For this review, take the finished solid that the model builds, in its own axes (mm). Give positions to 0.01 mm unless a question says otherwise; leave off trailing zeros. Loops run counter-clockwise (first coordinate to the right, second up) from the corner with the lowest first, then second, coordinate; pieces in that order, holes last. Notation, with made-up numbers: (30.25, 41) - (66.25, 41) arc R28 cw to (66.25, 69) - close; hole circle Ø5 at (-24, 14). An arc over 180 degrees is marked (long way). Put each result on its own line as item: value.
Autodesk Inventor part; units mm, degrees
ref_plane "YZ Plane" through (0, 0, 0) normal (1, 0, 0) x (0, 1, 0)
ref_plane "XZ Plane" through (0, 0, 0) normal (0, 1, 0) x (-1, 0, 0)
ref_plane "XY Plane" through (0, 0, 0) normal (0, 0, 1) x (1, 0, 0)
sketch "Sketch1" plane through (0, 0, 0) normal (0, 0, 1) x (1, 0, 0)
  line L0 (-101.9973, -32.9991) -> (101.9973, -32.9991)
  line L1 (-101.9973, 33.0009) -> (101.9973, 33.0009)
  line L2 (-103.9973, -30.9991) -> (-103.9973, 31.0009)
  line L3 (103.9973, 31.0009) -> (103.9973, -30.9991)
  arc A0 (-103.9973, -30.9991) -> (-101.9973, -32.9991) centre (-101.9973, -30.9991) ccw
  arc A1 (101.9973, -32.9991) -> (103.9973, -30.9991) centre (101.9973, -30.9991) ccw
  line L4 (103.9973, 31.0009) -> (103.9973, 33.0009)
  line L5 (101.9973, 33.0009) -> (103.9973, 33.0009)
  line L6 (-103.9973, 31.0009) -> (-103.9973, 33.0009)
  line L7 (-101.9973, 33.0009) -> (-103.9973, 33.0009)
  line L8 (57.998, 18.2189) -> (41.998, 18.2189)
  line L9 (41.998, 13.2189) -> (57.998, 13.2189)
  line L10 (-58.002, 18.2189) -> (-42.002, 18.2189)
  line L11 (-42.002, 13.2189) -> (-58.002, 13.2189)
  line L12 (32.998, 18.2189) -> (-33.002, 18.2189)
  line L13 (-33.002, 13.2189) -> (32.998, 13.2189)
  arc A2 (34.998, 16.2189) -> (32.998, 18.2189) centre (32.998, 16.2189) ccw
  arc A3 (-35.002, 15.2189) -> (-33.002, 13.2189) centre (-33.002, 15.2189) ccw
  arc A4 (-33.002, 18.2189) -> (-35.002, 16.2189) centre (-33.002, 16.2189) ccw
  arc A5 (-40.002, 16.2189) -> (-42.002, 18.2189) centre (-42.002, 16.2189) ccw
  arc A6 (-42.002, 13.2189) -> (-40.002, 15.2189) centre (-42.002, 15.2189) ccw
  arc A7 (-60.002, 15.2189) -> (-58.002, 13.2189) centre (-58.002, 15.2189) ccw
  arc A8 (-58.002, 18.2189) -> (-60.002, 16.2189) centre (-58.002, 16.2189) ccw
  arc A9 (39.998, 15.2189) -> (41.998, 13.2189) centre (41.998, 15.2189) ccw
  arc A10 (41.998, 18.2189) -> (39.998, 16.2189) centre (41.998, 16.2189) ccw
  arc A11 (59.998, 16.2189) -> (57.998, 18.2189) centre (57.998, 16.2189) ccw
  arc A12 (57.998, 13.2189) -> (59.998, 15.2189) centre (57.998, 15.2189) ccw
  arc A13 (32.998, 13.2189) -> (34.998, 15.2189) centre (32.998, 15.2189) ccw
  line L14 (59.998, 16.2189) -> (39.998, 16.2189)
  line L15 (39.998, 15.2189) -> (59.998, 15.2189)
  line L16 (34.998, 16.2189) -> (-35.002, 16.2189)
  line L17 (-35.002, 15.2189) -> (34.998, 15.2189)
  line L18 (-40.002, 16.2189) -> (-60.002, 16.2189)
  line L19 (-60.002, 15.2189) -> (-40.002, 15.2189)
  circle A14 centre (-59.9992, -3) radius 2
  circle A15 centre (59.9979, -3) radius 2
  line L20 (93.998, -24.9998) -> (93.998, -10.0006)
  line L21 (93.998, -10.0006) -> (98.998, -10.0006)
  line L22 (98.998, -24.9998) -> (98.998, -10.0006)
  line L23 (93.998, -24.9998) -> (98.998, -24.9998)
  line L24 (93.998, 9.9994) -> (93.998, 25.0009)
  line L25 (93.998, 25.0009) -> (98.998, 25.0009)
  line L26 (98.998, 9.9994) -> (98.998, 25.0009)
  line L27 (93.998, 9.9994) -> (98.998, 9.9994)
  line L28 (87.498, 20.0009) -> (57.498, 20.0009)
  line L29 (57.498, 20.0009) -> (57.498, 25.0009)
  line L30 (87.498, 25.0009) -> (57.498, 25.0009)
  line L31 (87.498, 20.0009) -> (87.498, 25.0009)
  line L32 (27.498, 20.0009) -> (-27.502, 20.0009)
  line L33 (-27.502, 20.0009) -> (-27.502, 25.0009)
  line L34 (27.498, 25.0009) -> (-27.502, 25.0009)
  line L35 (27.498, 20.0009) -> (27.498, 25.0009)
  line L36 (-57.502, 20.0009) -> (-87.502, 20.0009)
  line L37 (-87.502, 20.0009) -> (-87.502, 25.0009)
  line L38 (-57.502, 25.0009) -> (-87.502, 25.0009)
  line L39 (-57.502, 20.0009) -> (-57.502, 25.0009)
  line L40 (-99.002, 9.9994) -> (-99.002, 25.0009)
  line L41 (-99.002, 25.0009) -> (-94.002, 25.0009)
  line L42 (-94.002, 9.9994) -> (-94.002, 25.0009)
  line L43 (-99.002, 9.9994) -> (-94.002, 9.9994)
  line L44 (-99.002, -24.9998) -> (-99.002, -10.0006)
  line L45 (-99.002, -10.0006) -> (-94.002, -10.0006)
  line L46 (-94.002, -24.9998) -> (-94.002, -10.0006)
  line L47 (-99.002, -24.9998) -> (-94.002, -24.9998)
  point P0 (-85.2166, -15.942)
  point P1 (-103.9973, -32.9991)
  point P2 (103.9973, -32.9991)
  point P3 (59.998, 18.2189)
  point P4 (59.998, 13.2189)
  point P5 (-60.002, 16.2189)
  point P6 (59.998, 15.2189)
  point P7 (59.9979, -3)
extrude "Extrusion1" add sketch "Sketch1" along normal blind 5
properties part number "case bottom front" material "Nylon, molybdenum disulphide"
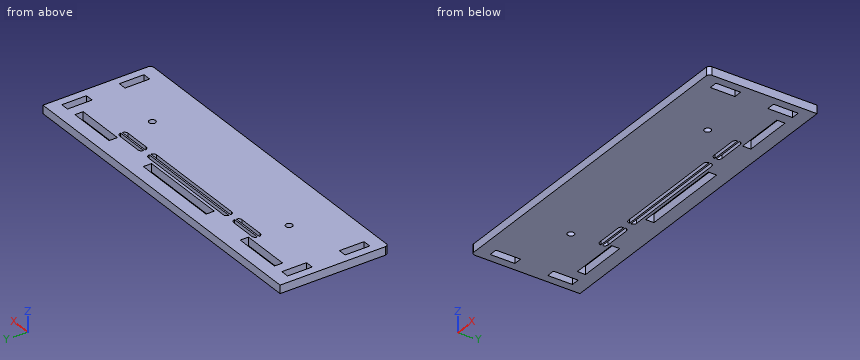
1) Wall thickness on line 1 (Y direction, x = -26, z = 2.7); line 2 (X direction, y = -14.5, z = 2.45); line 3 (Y direction, x = 29.5, z = 1.45): over which ranges is each line inside the solid? List them lowest first.
Geometry check:
line 1: y = -33 to 13.22, 15.22 to 16.22, 18.22 to 20, 25 to 33
line 2: x = -104 to -99, -94 to 94, 99 to 104
line 3: y = -33 to 13.22, 15.22 to 16.22, 18.22 to 33
2) Take a section at A-A on x = -7. State the section outline as (y, z) points.
Geometry check:
outline: (-33, 0) - (13.22, 0) - (13.22, 5) - (-33, 5) - close; (15.22, 0) - (16.22, 0) - (16.22, 5) - (15.22, 5) - close; (18.22, 0) - (20, 0) - (20, 5) - (18.22, 5) - close; (25, 0) - (33, 0) - (33, 5) - (25, 5) - close
3) Take a section at B-B on y = -3. State the section outline as (x, z) points.
Geometry check:
outline: (-104, 0) - (-62, 0) - (-62, 5) - (-104, 5) - close; (-58, 0) - (58, 0) - (58, 5) - (-58, 5) - close; (62, 0) - (104, 0) - (104, 5) - (62, 5) - close
4) Take a section at C-C on z = 3.4. State how many separate pieces and enclosed holes the cut face has, and give its area (3 significant figures).
Geometry check:
separate pieces: 1
enclosed holes: 15
area: 12,400 mm²
5) Insertion check: pin 1 Ø12 at (x, y) = (61.5, 24.5) entering from -Z. The pin has a flat end and moves straight along its axis. Give the tip position at first contact, or say it passes through.
Geometry check:
pin 1: stops at z = 0
